```python
from build123d import *

# Parameters (mm, degrees)
SKETCH1_R             = 30
BOSS_EXTRUDE1_DEPTH   = 2
BOSS_EXTRUDE2_START   = 4
SKETCH2_R             = 30
SKETCH2_R_2           = 25
BOSS_EXTRUDE2_DEPTH   = 4
BOSS_EXTRUDE3_REACH   = 44.849
SKETCH3_W             = 94
SKETCH3_H             = 40
SKETCH4_R             = 25
CUT_EXTRUDE1_DEPTH    = 4
SKETCH5_R             = 17.5
CUT_EXTRUDE2_DEPTH    = 56.901699437
FILLET1_R             = 6
M4X0_7_TAPPED_HOLE1_D = 3.3


with BuildPart() as part:
    # Sketch1 → Boss-Extrude1 (new body)
    with BuildSketch(Plane.XY):
        Circle(SKETCH1_R)
    extrude(amount=BOSS_EXTRUDE1_DEPTH)

    # Sketch2 → Boss-Extrude2 (add)
    with BuildSketch(Plane(origin=(0, 0, 0), x_dir=(-1, 0, 0), z_dir=(0, 0, -1)).offset(BOSS_EXTRUDE2_START)):
        Circle(SKETCH2_R)
        Circle(SKETCH2_R_2, mode=Mode.SUBTRACT)
    extrude(amount=-BOSS_EXTRUDE2_DEPTH)

    # Boss-Extrude3: up to this face of the body (flat: up to its plane)
    boss_extrude3_end = Plane(part.part.faces().sort_by_distance((0, 0, 2))[0])
    # Sketch3 → Boss-Extrude3 (add, up to the picked face)
    with BuildSketch(Plane(origin=(0, 0, -4), x_dir=(-1, 0, 0), z_dir=(0, 0, -1)), mode=Mode.PRIVATE) as boss_extrude3_sk1:
        Rectangle(SKETCH3_W, SKETCH3_H)
    boss_extrude3_tool1 = split(extrude(boss_extrude3_sk1.sketch, amount=-BOSS_EXTRUDE3_REACH, mode=Mode.PRIVATE), bisect_by=boss_extrude3_end, keep=Keep.BOTH, mode=Mode.PRIVATE)
    add(boss_extrude3_tool1.solids().sort_by(Axis((0, 0, -4), (0, 0, 1)))[0])

    # Sketch4 → Cut-Extrude1 (cut)
    with BuildSketch(Plane(origin=(0, 0, -4), x_dir=(-1, 0, 0), z_dir=(0, 0, -1))):
        Circle(SKETCH4_R)
    extrude(amount=-CUT_EXTRUDE1_DEPTH, mode=Mode.SUBTRACT)

    # Sketch5 → Cut-Extrude2 (cut, through all)
    with BuildSketch(Plane(origin=(0, 0, 0), x_dir=(-1, 0, 0), z_dir=(0, 0, -1))):
        Circle(SKETCH5_R)
    extrude(amount=-CUT_EXTRUDE2_DEPTH, mode=Mode.SUBTRACT)

    # Fillet1
    fillet1_edges = [part.edges().sort_by_distance(p)[0] for p in [
        (47, 0, 2),
        (34.680339887, -20, 2),
        (34.680339887, 20, 2),
        (0, 30, 2),
        (0, -30, 2),
        (-34.680339887, -20, 2),
        (-47, 0, 2),
        (-34.680339887, 20, 2),
    ]]
    fillet(fillet1_edges, radius=FILLET1_R - 0.0001)  # a hair under: the kernel refuses the full size

    # M4x0.7 Tapped Hole1 (through all)
    with Locations(Plane.XY.offset(2)):
        with Locations((-35, 10), (-35, -10), (35, 10), (35, -10)):
            Hole(M4X0_7_TAPPED_HOLE1_D / 2)


solid = part.part
```
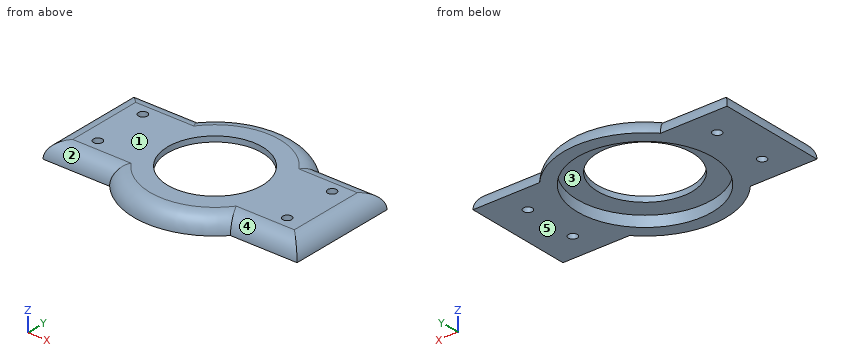
Check sheet for the modelled part. Datum: model origin and axes. Units: mm. Face numbers are marked on the shaded views. A direction names the side the tool comes from. Give positions to 0.01 mm unless a question says otherwise; leave off trailing zeros. Answer in a Markdown table with one row per item.
1) Cross-section at A-A (x = -35). Count the separate pieces of the cut face and the enclosed holes in it, plus the area to 3 significant figures.
Solutions:
| item | result |
|---|---|
| separate pieces | 3 |
| enclosed holes | 0 |
| area | 185 mm^2 |
2) Tool access check on the marked faces 1 and 2. Record the directions out of +Z, -Z, +X, -X, +Y, -Y that give a thin tool (end or side, any length) a straight path to the whole face; none if there is none.
Solutions:
| item | result |
|---|---|
| face 1 | +Z, +X, -X, +Y, -Y |
| face 2 | +Z, -X, -Y |
3) Thickness scan on line 1 (Z direction, x = 1.5, y = 17.5); line 2 (Y direction, x = 9, z = -1.5); line 3 (X direction, y = 5.5, z = -3.5). Record the ranges inside material, lowest first.
Solutions:
| item | result |
|---|---|
| line 1 | z = 0 to 2 |
| line 2 | y = -28.05 to -23.32, 23.32 to 28.05 |
| line 3 | x = -46.98 to -24.39, 24.39 to 46.98 |
4) Mould release check, pull along Y, two halves, no side actions. Record for the marked faces 3, 4 and 5: released by +Y, released by -Y, zero draft, split by the parting line, or undercut.
Solutions:
| item | result |
|---|---|
| face 3 | undercut |
| face 4 | released by -Y |
| face 5 | zero draft |
5) Depth check by flat-ended pin: pin 1 (2 mm diameter, centred on x = -31, z = 0, fed in from -Y); pin 2 (15 mm diameter, centred on x = -12, y = -7, fed in from -Z); pin 3 (2 mm diameter, centred on y = 17, z = 0.5, fed in from -X); pin 4 (4.5 mm diameter, centred on x = 35, y = -10, fed in from +Z). Enter the tip coordinate at first touch or a pass-through.
Solutions:
| item | result |
|---|---|
| pin 1 | stops at y = -19.2 |
| pin 2 | stops at z = 0 |
| pin 3 | stops at x = -45.87 |
| pin 4 | stops at z = 2 |
